from build123d import *

# Parameters (mm, degrees)
SKETCH2_W           = 10
SKETCH2_H           = 12
BOSS_EXTRUDE1_DEPTH = 26
BOSS_EXTRUDE2_DEPTH = 10


with BuildPart() as part:
    # Sketch2 → Boss-Extrude1 (new body)
    with BuildSketch(Plane(origin=(0, 0, 0), x_dir=(1, 0, 0), z_dir=(0, 1, 0))):
        Rectangle(SKETCH2_W, SKETCH2_H)
    extrude(amount=BOSS_EXTRUDE1_DEPTH)

    # Sketch3 → Boss-Extrude2 (add)
    with BuildSketch(Plane(origin=(0, 26, 0), x_dir=(1, 0, 0), z_dir=(0, 1, 0))):
        with BuildLine():
            ThreePointArc((1.5, 0), (1.060660172, 1.060660172), (0, 1.5))
            Line((0, 1.5), (0, -0.9))
            Line((0, -0.9), (1.2, -0.9))
            ThreePointArc((1.2, -0.9), (1.423024947, -0.474341649), (1.5, 0))
        make_face()
        with BuildLine():
            Line((0, -0.9), (0, 1.5))
            ThreePointArc((0, 1.5), (-1.341640786, 0.670820393), (-1.2, -0.9))
            Line((-1.2, -0.9), (0, -0.9))
        make_face()
    extrude(amount=BOSS_EXTRUDE2_DEPTH)


solid = part.part
Input: part model. Units: mm. Frame: model coordinates. A direction names the side the tool comes from. Coordinates: 2 decimals unless noted, no trailing zeros. Loops run counter-clockwise (first coordinate to the right, second up) from the corner with the lowest first, then second, coordinate; pieces in that order, holes last. Notation, with made-up numbers: (45.25, 48) - (73.25, 48) arc R27 ccw to (73.25, 72) - close; hole circle Ø3 at (44.25, -11.5). An arc over 180 degrees is marked (long way). Answer in a Markdown table with one row per item. Add a question column.
Item 1: Access query for faces 1 (the flat face through (5, 13, 0)), 2 (the flat face through (0, 31, 0.9)). Directions: +Z, -Z, +X, -X, +Y, -Y. A direction counts if a zero-diameter tool reaches every point of the face in a straight line with its end or side. Return the directions, or none.
Item 2: Line query: line 1 along Y through (x, z) = (-2.75, -1.75); line 2 along X through (y, z) = (29.5, -1). Output: solid intervals per line, ascending. Write a range as [from, to].
Item 3: Contact query for a flat-ended pin moving along its axis: P1, Ø1.2, axis at x = 0, y = 29, coming from the +Z side. Output: stop coordinate, or through.
Item 4: Section query A-A on z = -1. Return the cut outline in (x, y).
Item 5: Section query B-B on x = -0.5. Return the cut outline in (y, z), then the cut area to 3 significant figures.
Item 6: Section query D-D on x = 3.5. Return the cut outline in (y, z), then the cut area to 3 significant figures.
Item 7: Section query C-C on y = 34. Return the cut outline in (x, z), then the cut area to 3 significant figures.
Recorded:
| question | item | result |
|---|---|---|
| 1 | face 1 | +Z, -Z, +X, +Y, -Y |
| 1 | face 2 | +Z, +X, -X, +Y |
| 2 | line 1 | [0, 26] |
| 2 | line 2 | [-1.12, 1.12] |
| 3 | P1 | z = 0.9 |
| 4 | outline | (-5, 0) - (5, 0) - (5, 26) - (1.12, 26) - (1.12, 36) - (-1.12, 36) - (-1.12, 26) - (-5, 26) - close |
| 5 | outline | (0, -6) - (26, -6) - (26, -1.41) - (36, -1.41) - (36, 0.9) - (26, 0.9) - (26, 6) - (0, 6) - close |
| 5 | area | 335 mm^2 |
| 6 | outline | (0, -6) - (26, -6) - (26, 6) - (0, 6) - close |
| 6 | area | 312 mm^2 |
| 7 | outline | (-1.2, 0.9) arc R1.5 ccw (long way) to (1.2, 0.9) - close |
| 7 | area | 6.06 mm^2 |
